Verification items for the finished model (mm, model axes). Face numbers are marked on the shaded views. A direction names the side the tool comes from. Give positions to 0.01 mm unless a question says otherwise; leave off trailing zeros. Loops run counter-clockwise (first coordinate to the right, second up) from the corner with the lowest first, then second, coordinate; pieces in that order, holes last. Notation, with made-up numbers: M 47.25,-13 L 65.25,-13 A24 cw 65.25,15 Z; hole C 58.25,-27 d5. An arc over 180 degrees is marked long. Answer in a Markdown table with one row per item.
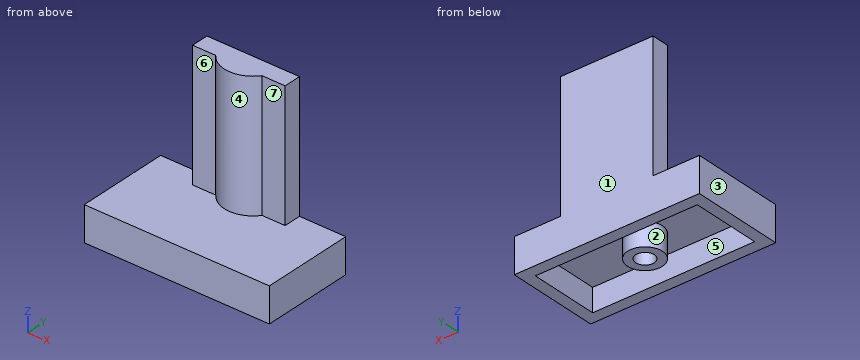
```python
from build123d import *

# Parameters (mm, degrees)
SKETCH1_W           = 16
SKETCH1_H           = 8
BOSS_EXTRUDE1_DEPTH = 3
SHELL3_T            = -1
SKETCH2_R           = 1.5
SKETCH2_R_2         = 0.8
BOSS_EXTRUDE2_DEPTH = 2
BOSS_EXTRUDE3_DEPTH = 11


with BuildPart() as part:
    # Sketch1 → Boss-Extrude1 (new body)
    with BuildSketch(Plane.XY):
        with Locations((-13.569515058, 18.04477027)):
            Rectangle(SKETCH1_W, SKETCH1_H)
    extrude(amount=BOSS_EXTRUDE1_DEPTH)

    # Shell3
    shell3_openings = [part.faces().sort_by_distance(p)[0] for p in [
        (-13.569515058, 18.04477027, 0),
    ]]
    offset(amount=SHELL3_T, openings=shell3_openings, kind=Kind.INTERSECTION)

    # Sketch2 → Boss-Extrude2 (add)
    with BuildSketch(Plane(origin=(0, 0, 2), x_dir=(-1, 0, 0), z_dir=(0, 0, -1))):
        with Locations((13.569515058, 18.04477027)):
            Circle(SKETCH2_R)
        with Locations((13.569515058, 18.04477027)):
            Circle(SKETCH2_R_2, mode=Mode.SUBTRACT)
    extrude(amount=BOSS_EXTRUDE2_DEPTH)

    # Sketch3 → Boss-Extrude3 (add)
    with BuildSketch(Plane.XY.offset(3)):
        with BuildLine():
            Line((-17.569515058, 22.04477027), (-17.569515058, 20.54477027))
            Line((-17.569515058, 20.54477027), (-15.569515058, 20.54477027))
            ThreePointArc((-15.569515058, 20.54477027), (-13.569515058, 19.54477027), (-11.569515058, 20.54477027))
            Line((-11.569515058, 20.54477027), (-9.569515058, 20.54477027))
            Line((-9.569515058, 20.54477027), (-9.569515058, 22.04477027))
            Line((-9.569515058, 22.04477027), (-17.569515058, 22.04477027))
        make_face()
    extrude(amount=BOSS_EXTRUDE3_DEPTH)


solid = part.part
```
Item 1: Sectioned sample at D-D (z = 12). Record the cut outline in (x, y), and give its area (3 significant figures).
Reported:
| item | result |
|---|---|
| outline | M -17.57,20.54 L -15.57,20.54 A2.5 ccw -11.57,20.54 L -9.57,20.54 L -9.57,22.04 L -17.57,22.04 Z |
| area | 14.8 mm^2 |
Item 2: Go/stop test with flat-tipped pins: pin 1 (0.5 mm diameter, centred on x = -13.5, y = 18, fed in from -Z); pin 2 (0.6 mm diameter, centred on x = -17, z = 10.5, fed in from -Y); pin 3 (0.8 mm diameter, centred on y = 21.5, z = 8.5, fed in from +X). Record where each tip stops, or that it passes through.
Reported:
| item | result |
|---|---|
| pin 1 | stops at z = 2 |
| pin 2 | stops at y = 20.54 |
| pin 3 | stops at x = -9.57 |
Item 3: Tool access check on the marked faces 4, 5, 6 and 7. Record the directions out of +Z, -Z, +X, -X, +Y, -Y that give a thin tool (end or side, any length) a straight path to the whole face; none if there is none.
Reported:
| item | result |
|---|---|
| face 4 | +Z, -Y |
| face 5 | -Z |
| face 6 | +Z, -X, -Y |
| face 7 | +Z, +X, -Y |
Item 4: Scan lines: L1, parallel to Y at x = -14.5, z = 1.5; L2, parallel to Y at x = -17.5, z = 8.75; L3, parallel to Z at x = -9.5, y = 19.5. Record each from-to range of solid material in increasing order. Write a range as [from, to].
Reported:
| item | result |
|---|---|
| L1 | y = [14.04, 15.04], [16.87, 19.22], [21.04, 22.04] |
| L2 | y = [20.54, 22.04] |
| L3 | z = [2, 3] |
Item 5: Sectioned sample at B-B (x = -9). Record the cut outline in (y, z).
Reported:
| item | result |
|---|---|
| outline | M 14.04,0 L 15.04,0 L 15.04,2 L 21.04,2 L 21.04,0 L 22.04,0 L 22.04,3 L 14.04,3 Z |
Item 6: Sectioned sample at A-A (z = 1.75). Record the cut outline in (x, y), and give its area (3 significant figures).
Reported:
| item | result |
|---|---|
| outline | M -21.57,14.04 L -5.57,14.04 L -5.57,22.04 L -21.57,22.04 Z; C -13.57,18.04 d3; hole M -20.57,15.04 L -6.57,15.04 L -6.57,21.04 L -20.57,21.04 Z; hole C -13.57,18.04 d1.6 |
| area | 49.1 mm^2 |
Item 7: Sectioned sample at C-C (y = 21.75). Record the cut outline in (x, z).
Reported:
| item | result |
|---|---|
| outline | M -21.57,0 L -5.57,0 L -5.57,3 L -9.57,3 L -9.57,14 L -17.57,14 L -17.57,3 L -21.57,3 Z |
Item 8: Release check for a two-part mould opening along X. For the marked faces 1, 2 and 3 record: released by +X, released by -X, zero draft, split by the parting line, or undercut.
Reported:
| item | result |
|---|---|
| face 1 | zero draft |
| face 2 | undercut |
| face 3 | released by -X |
